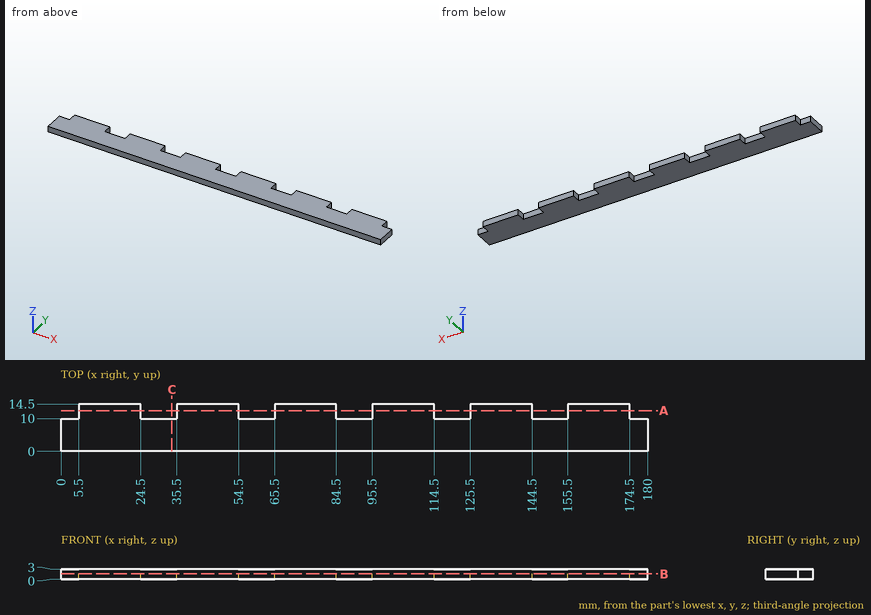
For this review, use the dimensioned drawing (mm, ordinates from the lowest corner) and the shaded views. Give positions to 0.01 mm unless a question says otherwise; leave off trailing zeros. Order: outer loops, then holes, each group sorted by start corner. A loop starts at its lowest first (then second) coordinate and runs counter-clockwise, first axis right, second up.
1) Wall thickness on line 1 (X direction, y = 12, z = 2.3); line 2 (Y direction, x = 34, z = 0.45): over which ranges is each line inside the solid? List them lowest first.
2) Insertion check: pin 1 (1.5 mm diameter, centred on y = 11, z = 1, fed in from -X); pin 2 (0.9 mm diameter, centred on x = 27.5, z = 2, fed in from +Y); pin 3 (1 mm diameter, centred on x = 84.5, z = 1.5, fed in from -Y); pin 4 (0.9 mm diameter, centred on y = 11.5, z = 2, fed in from +X). Each pin has a flat end and moves straight along its axis. Give the tip position at first contact, or say it passes through.
3) Take a section at A-A (y = 12.5). Give the boundary of the cut face in (x, z).
4) Take a section at B-B (z = 1.6). Give the boundary of the cut face in (x, y), then the cut area to 3 significant figures.
5) Take a section at C-C (x = 34). Give the boundary of the cut face in (y, z), then the cut area to 3 significant figures.
Derived:
1. line 1: x = 5.5 to 24.5, 35.5 to 54.5, 65.5 to 84.5, 95.5 to 114.5, 125.5 to 144.5, 155.5 to 174.5
1. line 2: y = 0 to 10
2. pin 1: stops at x = 5.5
2. pin 2: stops at y = 10
2. pin 3: stops at y = 0
2. pin 4: stops at x = 174.5
3. outline: (5.5, 0) - (24.5, 0) - (24.5, 3) - (5.5, 3) - close; (35.5, 0) - (54.5, 0) - (54.5, 3) - (35.5, 3) - close; (65.5, 0) - (84.5, 0) - (84.5, 3) - (65.5, 3) - close; (95.5, 0) - (114.5, 0) - (114.5, 3) - (95.5, 3) - close; (125.5, 0) - (144.5, 0) - (144.5, 3) - (125.5, 3) - close; (155.5, 0) - (174.5, 0) - (174.5, 3) - (155.5, 3) - close
4. outline: (0, 0) - (180, 0) - (180, 10) - (174.5, 10) - (174.5, 14.5) - (155.5, 14.5) - (155.5, 10) - (144.5, 10) - (144.5, 14.5) - (125.5, 14.5) - (125.5, 10) - (114.5, 10) - (114.5, 14.5) - (95.5, 14.5) - (95.5, 10) - (84.5, 10) - (84.5, 14.5) - (65.5, 14.5) - (65.5, 10) - (54.5, 10) - (54.5, 14.5) - (35.5, 14.5) - (35.5, 10) - (24.5, 10) - (24.5, 14.5) - (5.5, 14.5) - (5.5, 10) - (0, 10) - close
4. area: 2,310 mm2
5. outline: (0, 0) - (10, 0) - (10, 3) - (0, 3) - close
5. area: 30.0 mm2
